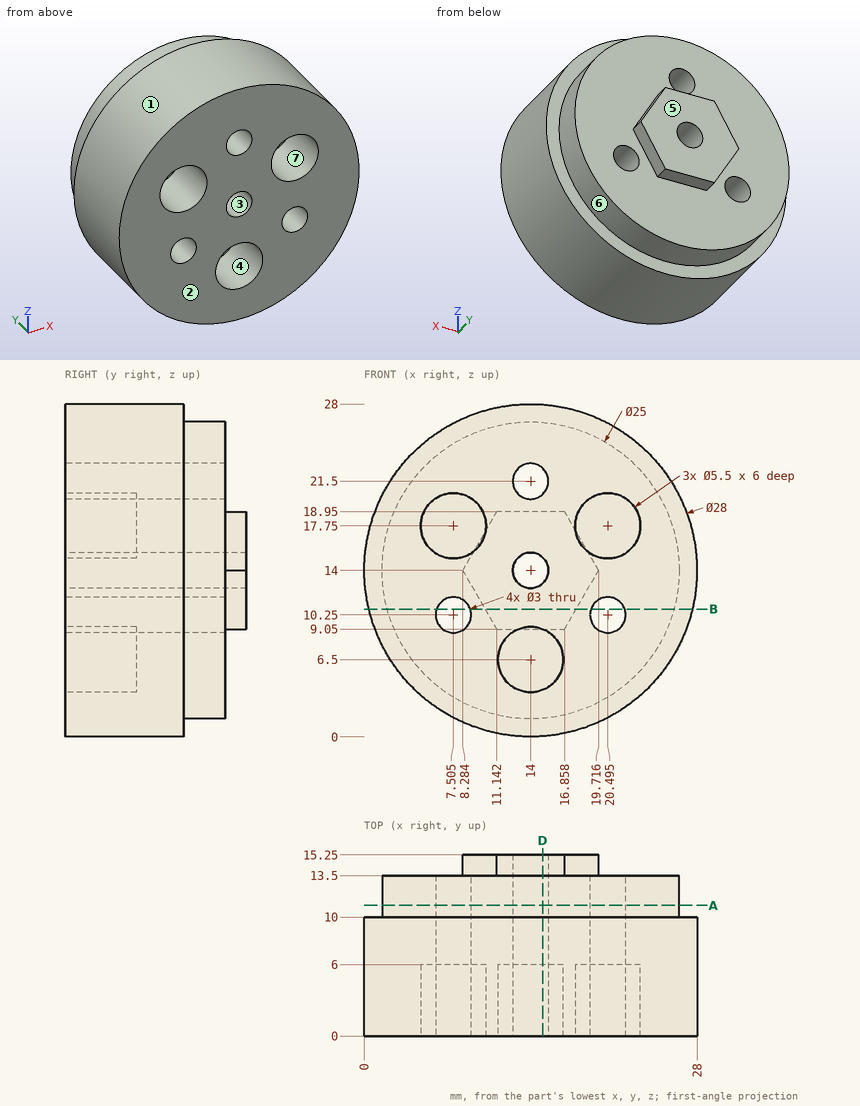
Design review of the part shown in the three views and the two pictorial views. Dimensions are in mm from the part's minimum x, y and z. A direction names the side the tool comes from. Round coordinates to 2 decimals unless told otherwise and drop trailing zeros. Loops run counter-clockwise (first coordinate to the right, second up) from the corner with the lowest first, then second, coordinate; pieces in that order, holes last.
(1) Wall thickness on line 1 along Z through (x, y) = (14, 9.25); line 2 along Z through (x, y) = (14, 11.25); line 3 along X through (y, z) = (1.2, 17.75) (1 decimal): over which ranges is each line inside the solid? List them lowest first.
Returned:
line 1: z = 0 to 12.5, 15.5 to 20, 23 to 28
line 2: z = 1.5 to 12.5, 15.5 to 20, 23 to 26.5
line 3: x = 0.5 to 4.8, 10.3 to 17.7, 23.2 to 27.5
(2) We need section A-A (y = 11). State how many separate pieces and enclosed holes the cut face has, plus the area to 3 significant figures.
Returned:
separate pieces: 1
enclosed holes: 4
area: 463 mm2
(3) Tool access review of the marked faces 5, 6 and 7: name each direction out of +Z, -Z, +X, -X, +Y, -Y from which nothing blocks a thin tool from reaching the whole face with its end or side.
Returned:
face 5: +Z, -Z, +X, -X, +Y
face 6: +Y
face 7: -Y
(4) Clearance check with flat-ended pins moving along their axes: P1, Ø4, axis at x = 20.5, z = 10.25, coming from the +Y side; P2, Ø4, axis at y = 10.5, z = 7, coming from the -X side; P3, Ø1.9, axis at x = 15.5, y = 15, coming from the -Z side. State where each tip first meets the part, or that it passes through.
Returned:
P1: stops at y = 13.5
P2: stops at x = 0.95
P3: stops at z = 9.05
(5) We need section D-D (x = 15). Give the boundary of the cut face in (y, z), plus the area to 3 significant figures.
Returned:
outline: (0, 0.04) - (10, 0.04) - (10, 1.54) - (13.5, 1.54) - (13.5, 9.05) - (15.25, 9.05) - (15.25, 12.88) - (0, 12.88) - (0, 9.06) - (6, 9.06) - (6, 3.94) - (0, 3.94) - close; (0, 15.12) - (15.25, 15.12) - (15.25, 18.95) - (13.5, 18.95) - (13.5, 20.38) - (0, 20.38) - close; (0, 22.62) - (13.5, 22.62) - (13.5, 26.46) - (10, 26.46) - (10, 27.96) - (0, 27.96) - close
area: 289 mm2
(6) We need section B-B (z = 10.75). Give the boundary of the cut face in (x, y).
Returned:
outline: (0.38, 0) - (6.09, 0) - (6.09, 13.5) - (1.93, 13.5) - (1.93, 10) - (0.38, 10) - close; (8.92, 0) - (19.08, 0) - (19.08, 13.5) - (17.84, 13.5) - (17.84, 15.25) - (10.16, 15.25) - (10.16, 13.5) - (8.92, 13.5) - close; (21.91, 0) - (27.62, 0) - (27.62, 10) - (26.07, 10) - (26.07, 13.5) - (21.91, 13.5) - close
(7) Mouldability with a two-part tool opening along Z and no side actions: class the marked faces 1, 2, 3 and 4 as released by +Z, released by -Z, zero draft, split by the parting line, or undercut.
Returned:
face 1: split by the parting line
face 2: zero draft
face 3: undercut
face 4: undercut
